Read the model definition and answer for the solid it produces. Units are mm, in the model's axes. Round coordinates to 2 decimals unless told otherwise and drop trailing zeros. Order: outer loops, then holes, each group sorted by start corner. A loop starts at its lowest first (then second) coordinate and runs counter-clockwise, first axis right, second up. Notation, with made-up numbers: (-9.75, 59) - (14.25, 59) arc R7 ccw to (14.25, 69) - close; hole circle Ø3 at (30.5, 55.25). An arc over 180 degrees is marked (long way). Put each result on its own line as item: value. Start each with the question number.
Q1. Find the intervals of material crossed by line 1 along X through (y, z) = (2.05, -69); line 2 along X through (y, z) = (2.25, -156); line 3 along Z through (x, y) = (72, 1.55), in increasing order. Write a range as from..to.
Q2. Section C-C on x = 16.5 is taken. Give the vertices of the cut face in (y, z).
Q3. Each of these flat-tipped pins is pushed along its axis until it touches: pin 1 Ø10 at (x, z) = (71, -143.5) entering from +Y; pin 2 Ø0.9 at (y, z) = (1, -3.5) entering from +X; pin 3 Ø1.5 at (x, y) = (-95, 1) entering from +Z. Where does it stop, or does it pass through?
Q4. Section A-A on z = -17.5 is taken. Give the vertices of the cut face in (x, y), then the cut area to 3 significant figures.
Q5. Section B-B on y = 0.5 is taken. State how many separate pieces and enclosed holes the cut face has, then the cut area to 3 significant figures.
from build123d import *

# Parameters (mm, degrees)
SKETCH1_W           = 225.24
SKETCH1_H           = 169.09
BOSS_EXTRUDE1_DEPTH = 3
SKETCH2_W           = 63.5
SKETCH2_H           = 154.09
SKETCH2_W_2         = 45.24
SKETCH2_H_2         = 10
SKETCH2_W_3         = 25.01
CUT_EXTRUDE1_DEPTH  = 204.183888387
SKETCH3_W           = 5
SKETCH3_H           = 3
BOSS_EXTRUDE2_DEPTH = 17
SKETCH4_W           = 5
SKETCH4_H           = 3
BOSS_EXTRUDE3_DEPTH = 17
SKETCH5_W           = 6
SKETCH5_H           = 159.09
CUT_EXTRUDE2_DEPTH  = 204.183888387


with BuildPart() as part:
    # Sketch1 → Boss-Extrude1 (new body)
    with BuildSketch(Plane(origin=(0, 0, 0), x_dir=(1, 0, 0), z_dir=(0, 1, 0))):
        with Locations((0, 84.545)):
            Rectangle(SKETCH1_W, SKETCH1_H)
    extrude(amount=BOSS_EXTRUDE1_DEPTH)

    # Sketch2 → Cut-Extrude1 (cut, through all)
    with BuildSketch(Plane(origin=(0, 0, 0), x_dir=(1, 0, 0), z_dir=(0, 1, 0))):
        Polygon((36.63, 25), (36.63, 155), (77.38, 155), (77.38, 169.09), (89.38, 169.09), (89.38, 25), align=None)
        Polygon((-100.99, 169.09), (-89, 169.09), (-89, 155), (-56.87, 155), (-56.87, 25), (-100.99, 25), align=None)
        with Locations((-10.12, 92.045)):
            Rectangle(SKETCH2_W, SKETCH2_H)
        with Locations((90, 5)):
            Rectangle(SKETCH2_W_2, SKETCH2_H_2)
        with Locations((-100.115, 5)):
            Rectangle(SKETCH2_W_3, SKETCH2_H_2)
    extrude(amount=CUT_EXTRUDE1_DEPTH, mode=Mode.SUBTRACT)

    # Sketch3 → Boss-Extrude2 (add)
    with BuildSketch(Plane.ZY.offset(-89.38)):
        with Locations((-152.5, 1.5)):
            Rectangle(SKETCH3_W, SKETCH3_H)
    extrude(amount=BOSS_EXTRUDE2_DEPTH)

    # Sketch4 → Boss-Extrude3 (add)
    with BuildSketch(Plane(origin=(-100.99, 0, 0), x_dir=(0, 0, -1), z_dir=(1, 0, 0))):
        with Locations((152.5, 1.5)):
            Rectangle(SKETCH4_W, SKETCH4_H)
    extrude(amount=BOSS_EXTRUDE3_DEPTH)

    # Sketch5 → Cut-Extrude2 (cut, through all)
    with BuildSketch(Plane(origin=(0, 3, 0), x_dir=(1, 0, 0), z_dir=(0, 1, 0))):
        with Locations((109.62, 89.545)):
            Rectangle(SKETCH5_W, SKETCH5_H)
    extrude(amount=-CUT_EXTRUDE2_DEPTH, mode=Mode.SUBTRACT)


solid = part.part
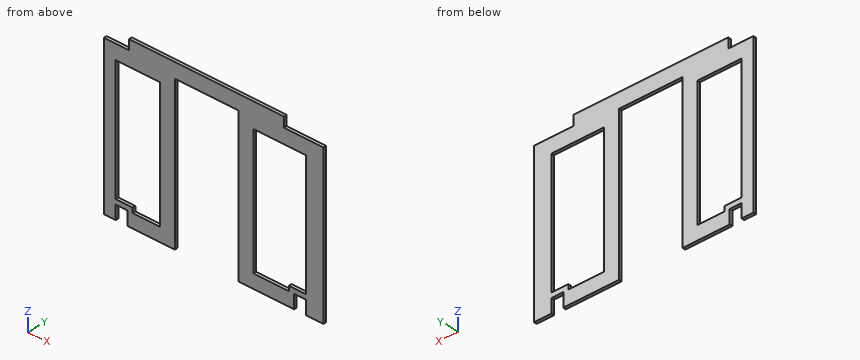
Findings:
1. line 1: -112.62..-100.99, -56.87..-41.87, 21.63..36.63, 89.38..106.62
1. line 2: -112.62..-100.99, -89..-41.87, 21.63..77.38, 89.38..106.62
1. line 3: -169.09..-155, -25..-10
2. outline: (0, -15) - (3, -15) - (3, 0) - (0, 0) - close
3. pin 1: through
3. pin 2: x = 67.38
3. pin 3: z = -10
4. outline: (-112.62, 0) - (-41.87, 0) - (-41.87, 3) - (-112.62, 3) - close; (21.63, 0) - (106.62, 0) - (106.62, 3) - (21.63, 3) - close
4. area: 467 mm2
5. separate pieces: 1
5. enclosed holes: 2
5. area: 13,900 mm2
